Autodesk Inventor part; units mm, degrees
ref_plane "YZ Plane" through (0, 0, 0) normal (1, 0, 0) x (0, 1, 0)
ref_plane "XZ Plane" through (0, 0, 0) normal (0, 1, 0) x (-1, 0, 0)
ref_plane "XY Plane" through (0, 0, 0) normal (0, 0, 1) x (1, 0, 0)
sketch "Sketch1" plane through (0, 0, 0) normal (0, 0, 1) x (1, 0, 0)
  circle A0 centre (0, 0) radius 2.413
  dimension "d0" = 4.826
extrude "Extrusion1" add sketch "Sketch1" along normal blind 9.525
sketch "Sketch2" plane through (0, 0, 0) normal (0, 1, 0) x (-1, 0, 0)
  line L0 (0, 0) -> (0, -2.5654)
  line L1 (0, 0) -> (4.5085, 0)
  line L2 (0, -2.5654) -> (2.032, -2.5654)
  line L3 (4.5085, 0) -> (4.5085, 4.071) construction
  arc A0 (4.5791, -0.105) -> (4.5085, 0) centre (4.5085, -0.0762) ccw
  arc A1 (2.032, -2.5654) -> (4.5791, -0.105) centre (0.5168, 1.5517) ccw
  line L4 (4.5847, 0.6553) -> (4.5847, -0.0762) construction
  dimension "d3" = 2.5654
  dimension "d6" = 2.032
  dimension "d12" = 4.5847
  dimension "d18" = 0.0762
revolve "Revolution1" add sketch "Sketch2" angle 360 about axis through (0, 0, 0) along (0, 0, -1)
sketch "Sketch3" plane through (0, 0, -2.5654) normal (0, 0, -1) x (-1, 0, 0)
  circle A0 centre (0, 0) radius 2.032
  line L0 (-0.9165, 1.5875) -> (0.9165, 1.5875)
  line L1 (0.9165, 1.5875) -> (1.8331, 0)
  line L2 (1.8331, 0) -> (0.9165, -1.5875)
  line L3 (0.9165, -1.5875) -> (-0.9165, -1.5875)
  line L4 (-0.9165, -1.5875) -> (-1.8331, 0)
  line L5 (-1.8331, 0) -> (-0.9165, 1.5875)
  dimension "d8" = 3.175
extrude "Extrusion2" cut sketch "Sketch3" against normal blind 1.5875 contours L0 L1 L2 L3 L4 L5
chamfer "Chamfer1" distance 0.508 angle 45 1 edges at (-2.413, 0, 9.525)
thread "Thread1"
properties part number "10-32 BHCS x375" material "Steel"
CAD build for the part. Positions are in the model's coordinates, mm. A direction names the side the tool comes from. Round coordinates to 2 decimals unless told otherwise and drop trailing zeros. Write each loop counter-clockwise with the first axis right and the second up, starting at its lowest first coordinate (ties: lowest second). Pieces come first, ordered by that corner, then holes.
(1) Mould opens along X. For faces 1 (the face through (0, 0, 9.525)), 2 (the face through (0, 1.588, -2)), 3 (the face through (-1.915, 1.468, 4.445)) say: pulls with the +X half, pulls with the -X half, needs draft (parallel to the pull), parting line crosses it, or undercut.
(2) Slice it at A-A, the plane z = 5.5. Write the cut outline in (x, y).
(3) Drop flat-ended pins along their axis: P1, Ø2, axis at x = 0, z = 6.5, coming from the +Y side; P2, Ø1.7, axis at x = 0.5, z = -2, coming from the +Y side; P3, Ø1.7, axis at x = -0.5, z = -1.5, coming from the -Y side; P4, Ø1.6, axis at x = 0, y = -1, coming from the -Z side. Give the stop position or say it passes through.
(4) Probe line 1 along Z through (x, y) = (0.75, -0.25) (3 decimals); line 2 along X through (y, z) = (1.5, 4.75); line 3 along Z through (x, y) = (4.25, -0.5). List the from-to ranges inside material, lowest first.
(5) 3-axis set-ups, long thin cutter, end or side, ignore diameter. For faces 4 (the face through (-1.381, -0.783, -1.783)), 5 (the face through (-2, -2, 0)): which of +Z, -Z, +X, -X, +Y, -Y reach the whole face in a straight line?
From the geometry:
1. face 1: needs draft
1. face 2: undercut
1. face 3: parting line crosses it
2. outline: circle Ø4.83 at (0, 0)
3. P1: stops at y = 2.41
3. P2: stops at y = 3.95
3. P3: stops at y = -4.29
3. P4: stops at z = -2.57
4. line 1: z = -0.978 to 9.525
4. line 2: x = -1.89 to 1.89
4. line 3: z = -0.7 to 0
5. face 4: -Z
5. face 5: +Z
